Design review of the part built by this model. Coordinates are the model's own, in mm. A direction names the side the tool comes from. Coordinates: 2 decimals unless noted, no trailing zeros. Order: outer loops, then holes, each group sorted by start corner. A loop starts at its lowest first (then second) coordinate and runs counter-clockwise, first axis right, second up. Notation, with made-up numbers: M 11.25,37.25 L 35.25,37.25 A26 ccw 35.25,61.25 Z; hole C -35,6 d7. An arc over 180 degrees is marked long. Answer in a Markdown table with one row per item.
from build123d import *

# Parameters (mm, degrees)
SKETCH1_W           = 27.2
SKETCH1_H           = 52
BOSS_EXTRUDE1_DEPTH = 2
SKETCH2_W           = 0.5
SKETCH2_H           = 52
CUT_EXTRUDE1_DEPTH  = 1
SKETCH3_W           = 0.5
SKETCH3_H           = 52
CUT_EXTRUDE2_DEPTH  = 1
SKETCH4_W           = 0.5
SKETCH4_H           = 2
CUT_EXTRUDE3_DEPTH  = 4.5
SKETCH5_W           = 0.5
SKETCH5_H           = 2
CUT_EXTRUDE4_DEPTH  = 4.5
SKETCH6_W           = 4.2
SKETCH6_H           = 1
CUT_EXTRUDE5_DEPTH  = 4.5
SKETCH9_W           = 27.2
SKETCH9_H           = 1
BOSS_EXTRUDE3_DEPTH = 4
FILLET1_R           = 2


with BuildPart() as part:
    # Sketch1 → Boss-Extrude1 (new body)
    with BuildSketch(Plane.XY):
        with Locations((13.6, 26)):
            Rectangle(SKETCH1_W, SKETCH1_H)
    extrude(amount=BOSS_EXTRUDE1_DEPTH)

    # Sketch2 → Cut-Extrude1 (cut)
    with BuildSketch(Plane.XY.offset(2)):
        with Locations((0.25, 26)):
            Rectangle(SKETCH2_W, SKETCH2_H)
    extrude(amount=-CUT_EXTRUDE1_DEPTH, mode=Mode.SUBTRACT)

    # Sketch3 → Cut-Extrude2 (cut)
    with BuildSketch(Plane.XY.offset(2)):
        with Locations((26.95, 26)):
            Rectangle(SKETCH3_W, SKETCH3_H)
    extrude(amount=-CUT_EXTRUDE2_DEPTH, mode=Mode.SUBTRACT)

    # Sketch4 → Cut-Extrude3 (cut)
    with BuildSketch(Plane(origin=(0, 52, 0), x_dir=(1, 0, 0), z_dir=(0, 1, 0))):
        with Locations((10.75, -1)):
            Rectangle(SKETCH4_W, SKETCH4_H)
    extrude(amount=-CUT_EXTRUDE3_DEPTH, mode=Mode.SUBTRACT)

    # Sketch5 → Cut-Extrude4 (cut)
    with BuildSketch(Plane(origin=(0, 52, 0), x_dir=(1, 0, 0), z_dir=(0, 1, 0))):
        with Locations((15.45, -1)):
            Rectangle(SKETCH5_W, SKETCH5_H)
    extrude(amount=-CUT_EXTRUDE4_DEPTH, mode=Mode.SUBTRACT)

    # Sketch6 → Cut-Extrude5 (cut)
    with BuildSketch(Plane(origin=(0, 52, 0), x_dir=(1, 0, 0), z_dir=(0, 1, 0))):
        with Locations((13.1, -0.5)):
            Rectangle(SKETCH6_W, SKETCH6_H)
    extrude(amount=-CUT_EXTRUDE5_DEPTH, mode=Mode.SUBTRACT)

    # Sketch9 → Boss-Extrude3 (add)
    with BuildSketch(Plane(origin=(0, 0, 0), x_dir=(-1, 0, 0), z_dir=(0, 0, -1))):
        with Locations((-13.6, 0.5)):
            Rectangle(SKETCH9_W, SKETCH9_H)
    extrude(amount=-BOSS_EXTRUDE3_DEPTH)

    # Fillet1
    fillet1_edges = [part.edges().sort_by_distance(p)[0] for p in [
        (13.6, 0, 0),
    ]]
    fillet(fillet1_edges, radius=FILLET1_R)


solid = part.part
(1) Add section A-A, the plane y = 31.5. Give the boundary of the cut face in (x, z).
Return value:
| item | result |
|---|---|
| outline | M 0,0 L 27.2,0 L 27.2,1 L 26.7,1 L 26.7,2 L 0.5,2 L 0.5,1 L 0,1 Z |
(2) Add section C-C, the plane z = 3.05. Give the boundary of the cut face in (x, y).
Return value:
| item | result |
|---|---|
| outline | M 0,0 L 27.2,0 L 27.2,1 L 0,1 Z |
(3) Add section B-B, the plane x = 6. Give the boundary of the cut face in (y, z), and give its area (3 significant figures).
Return value:
| item | result |
|---|---|
| outline | M 0,2 A2 ccw 2,0 L 52,0 L 52,2 L 1,2 L 1,4 L 0,4 Z |
| area | 105 mm2 |
(4) For faces 1 (the flat face through (13, 50, 1)), 2 (the flat face through (15.7, 50, 1)), 3 (the flat face through (0, 24, 0.7)), 4 (the flat face through (26.7, 26.1, 1.5)), list the 3-axis set-ups (+Z, -Z, +X, -X, +Y, -Y) from which the entire face can be reached by the end or side of a thin tool; tool diameter is ignored.
Return value:
| item | result |
|---|---|
| face 1 | -Z, +Y |
| face 2 | +Z, -Z, +Y |
| face 3 | +Z, -Z, -X, +Y, -Y |
| face 4 | +Z, +X, +Y |
(5) Insertion check: pin 1 Ø0.9 at (x, z) = (19, 3) entering from +Y; pin 2 Ø10 at (x, y) = (21.5, 30.5) entering from +Z; pin 3 Ø2 at (y, z) = (7, 2.5) entering from +X. Each pin has a flat end and moves straight along its axis. Give the tip position at first contact, or say it passes through.
Return value:
| item | result |
|---|---|
| pin 1 | stops at y = 1 |
| pin 2 | stops at z = 2 |
| pin 3 | stops at x = 26.7 |
(6) Draft analysis for pull direction X (two halves, no side actions). For faces 5 (the flat face through (13, 27, 2)), 6 (the flat face through (15.2, 49.8, 1.5)), 7 (the flat face through (27.2, 24, 0.7)), 8 (the flat face through (10.5, 50, 1)), state which applies: pulls with the +X half, pulls with the -X half, needs draft (parallel to the pull), parting line crosses it, or undercut.
Return value:
| item | result |
|---|---|
| face 5 | needs draft |
| face 6 | undercut |
| face 7 | pulls with the +X half |
| face 8 | undercut |
(7) For line 1 along X through (y, z) = (48, 0.95); line 2 along Z through (x, y) = (8, 30.5); line 3 along X through (y, z) = (29, 1.3), list the stretches that pass through material, from the lowest coordinate up. Write a range as from..to.
Return value:
| item | result |
|---|---|
| line 1 | x = 0..10.5, 15.7..27.2 |
| line 2 | z = 0..2 |
| line 3 | x = 0.5..26.7 |
